Geometry: final body of the model. Coordinates: model frame, mm. A direction names the side the tool comes from. Coordinates: 2 decimals unless noted, no trailing zeros. Write each loop counter-clockwise with the first axis right and the second up, starting at its lowest first coordinate (ties: lowest second). Pieces come first, ordered by that corner, then holes. Notation, with made-up numbers: M 81.5,16.25 L 90.5,16.25 A30 cw 90.5,44.25 Z; hole C -33.5,21 d10. An arc over 180 degrees is marked long. Write item = value, one per line. Start each with the question number.
Item 1: Section C-C on x = 22. Output: boundary loops of the cut face in (y, z), plus the area to 3 significant figures.
Item 2: Ray query, L1, parallel to Y at x = 2.5, z = 2; L2, parallel to X at y = 4.25, z = 5; L3, parallel to X at y = 1.5, z = 6. Return the intervals inside material, ascending. Write a range as [from, to].
Item 3: Pull-direction query (X, two-part tool) for faces 4 (the flat face through (2, 5.1, 4)), 5 (the flat face through (3, 18.987, 4)), 6 (the flat face through (6.341, 21, 4)); classes: +X half, -X half, draft (parallel to the pull), parting line (faces both ways), or undercut.
Item 4: First-contact query: pin 1 Ø2 at (x, z) = (15.5, 2) entering from -Y; pin 2 Ø1 at (x, y) = (24.5, 13.5) entering from +Z; pin 3 Ø0.7 at (y, z) = (1.5, 1.5) entering from +X; pin 4 Ø3.5 at (x, z) = (1, 4.5) entering from +Y. Flat tips, straight axial feed; report the tip coordinate or a pass-through.
Item 5: Reachability of faces 1 (the flat face through (1, -0.237, 4)), 2 (the flat face through (8.071, 1, 2)), 3 (the flat face through (1, 3, 3.35)) from +Z, -Z, +X, -X, +Y, -Y: full face, straight path, thin tool, end or side. Return the list, or none.
Item 6: Section A-A on z = 6.75. Output: boundary loops of the cut face in (x, y).
from build123d import *

# Parameters (mm, degrees)
PAD_DEPTH     = 0.1
SKETCH001_W   = 2.992089
SKETCH001_H   = 0.5
SKETCH001_W_2 = 2.718208
SKETCH001_H_2 = 0.25
PAD001_DEPTH  = 8
SKETCH003_W   = 3
SKETCH003_H   = 2.3
SKETCH003_W_2 = 2
SKETCH003_H_2 = 4.980278
SKETCH003_W_3 = 0.25
SKETCH003_H_3 = 5.1
PAD002_DEPTH  = 3.25
SKETCH004_R   = 0.9
PAD003_DEPTH  = 0.2


with BuildPart() as part:
    # Sketch → Pad (new body)
    with BuildSketch(Plane.XY):
        Polygon((0, 0), (0, 19), (6.33, 19), (6.33, 23), (7.95, 25.283769), (13.95, 25.283769), (15.57, 23), (15.57, 19), (27.57, 19), (27.57, 0), align=None)
    extrude(amount=PAD_DEPTH)

    # Sketch001 → Pad001 (new body)
    with BuildSketch(Plane.XY.offset(0.1)):
        Polygon((0, 18.987083), (0, 0), (-0.247297, 0), (-0.247297, 19.200211), (6.090689, 19.200211), (6.090689, 23.019194), (6.340689, 23.019194), (6.340689, 18.987083), align=None)
        Polygon((5.45, 5.1), (8.25, 5.1), (8.25, 0), (8.532358, 0), (8.532358, 5.35), (5.45, 5.35), align=None)
        Polygon((2.75, 0), (4.785295, 1.712651), (4.84968, 1.636137), (2.814385, -0.076515), align=None)
        with Locations((1.535533, 5.35)):
            Rectangle(SKETCH001_W, SKETCH001_H)
        with Locations((1.380876, -0.111513)):
            Rectangle(SKETCH001_W_2, SKETCH001_H_2)
    extrude(amount=PAD001_DEPTH)

    # Sketch003 → Pad002 (new body)
    with BuildSketch(Plane.XY.offset(0.1)):
        with Locations((6.555456, 3.832422)):
            Rectangle(SKETCH003_W, SKETCH003_H)
        with Locations((6.570963, 1.391803)):
            Rectangle(SKETCH003_W, SKETCH003_H)
        with Locations((1.036032, 2.552082)):
            Rectangle(SKETCH003_W_2, SKETCH003_H_2)
        with Locations((8.375, 2.55)):
            Rectangle(SKETCH003_W_3, SKETCH003_H_3)
        Polygon((2.75, 0), (4.785295, 1.712651), (4.84968, 1.636137), (2.814385, -0.076515), align=None)
    extrude(amount=PAD002_DEPTH)

    # Sketch004 → Pad003 (new body)
    with BuildSketch(Plane(origin=(5.070963, 0, 0), x_dir=(0, -1, 0), z_dir=(-1, 0, 0))):
        with Locations((-3.804629, 1.627155)):
            Circle(SKETCH004_R)
        with Locations((-1.376705, 1.679936)):
            Circle(SKETCH004_R)
    extrude(amount=PAD003_DEPTH)


solid = part.part
Responses:
q1.outline = M 0,0 L 19,0 L 19,0.1 L 0,0.1 Z
q1.area = 1.90 mm²
q2.L1 = [-0.24, 0.01], [5.1, 5.6], [18.99, 19.2]
q2.L2 = [-0.25, 0], [8.25, 8.53]
q2.L3 = [-0.25, 0], [4.53, 4.69], [8.25, 8.53]
q3.face_4 = undercut
q3.face_5 = draft
q3.face_6 = +X half
q4.pin_1 = through
q4.pin_2 = 0.1
q4.pin_3 = 8.53
q4.pin_4 = 19.2
q5.face_1 = +Z, -Z, +X, -X, -Y
q5.face_2 = +Z, -Y
q5.face_3 = +Z
q6.outline = M -0.25,0 L 0,0 L 0,18.99 L 6.34,18.99 L 6.34,23.02 L 6.09,23.02 L 6.09,19.2 L -0.25,19.2 Z; M 0.02,-0.24 L 2.74,-0.24 L 2.74,0.01 L 0.02,0.01 Z; M 0.04,5.1 L 3.03,5.1 L 3.03,5.6 L 0.04,5.6 Z; M 2.75,0 L 2.81,-0.08 L 4.85,1.64 L 4.79,1.71 Z; M 5.45,5.1 L 8.25,5.1 L 8.25,0 L 8.53,0 L 8.53,5.35 L 5.45,5.35 Z
